The listing builds one solid part. Answer for the finished solid, in the listing's coordinates (mm). Round coordinates to 2 decimals unless told otherwise and drop trailing zeros. Loops run counter-clockwise (first coordinate to the right, second up) from the corner with the lowest first, then second, coordinate; pieces in that order, holes last. Notation, with made-up numbers: M -37,41 L 8,41 A15 cw 8,45 Z; hole C 80.5,76 d11. An arc over 180 degrees is marked long. Answer as a JSON object with one key per item and string values.
```python
from build123d import *

# Parameters (mm, degrees)
CORTAR_EXTRUIR1_DEPTH      = 11.998522628
CORTAR_EXTRUIR1_DEPTH_BACK = 11.998522628
CROQUIS2_R                 = 3
CORTAR_EXTRUIR2_DEPTH      = 11.998522628
CORTAR_EXTRUIR2_DEPTH_BACK = 11.998522628
CROQUIS3_W                 = 1.096650784
CROQUIS3_H                 = 12.7
REDONDEO1_R                = 0.25
CHAFL_N1_SIZE              = 0.5


with BuildPart() as part:
    # Croquis1 → Revolución1 (revolve)
    with BuildSketch(Plane.XY):
        with BuildLine():
            Line((0, 6.35), (0, -6.35))
            ThreePointArc((0, -6.35), (-6.35, 0), (0, 6.35))
        make_face()
    revolve(axis=Axis((0, 6.35, 0), (0, -1, 0)))

    # Croquis2 → Cortar-Extruir1 (cut, two sides: drawn at the far end of the back side and taken through both)
    with BuildSketch(Plane.XY.offset(-CORTAR_EXTRUIR1_DEPTH_BACK)):
        with Locations(Location((0, 0, 0), (0, 0, 180))):
            Circle(CROQUIS2_R)
    extrude(amount=CORTAR_EXTRUIR1_DEPTH + CORTAR_EXTRUIR1_DEPTH_BACK, mode=Mode.SUBTRACT)

    # Croquis3 → Cortar-Extruir2 (cut, two sides: drawn at the far end of the back side and taken through both)
    with BuildSketch(Plane(origin=(0, 0, 0), x_dir=(0, 0, -1), z_dir=(1, 0, 0)).offset(-CORTAR_EXTRUIR2_DEPTH_BACK)):
        with Locations((5.048325392, 0)):
            Rectangle(CROQUIS3_W, CROQUIS3_H)
        with Locations((-5.048325392, 0)):
            Rectangle(CROQUIS3_W, CROQUIS3_H)
    extrude(amount=CORTAR_EXTRUIR2_DEPTH + CORTAR_EXTRUIR2_DEPTH_BACK, mode=Mode.SUBTRACT)

    # Redondeo1
    redondeo1_edges = [part.edges().sort_by_distance(p)[0] for p in [
        (0, -4.480234369, 4.5),
        (0, 4.480234369, -4.5),
    ]]
    fillet(redondeo1_edges, radius=REDONDEO1_R)

    # Chaflán1
    chafl_n1_edges = [part.edges().sort_by_distance(p)[0] for p in [
        (3, 0, 4.5),
        (3, 0, -4.5),
    ]]
    chamfer(chafl_n1_edges, length=CHAFL_N1_SIZE)


solid = part.part
```
Item 1: The part is cut by section B-B (x = 5.75). Give the vertices of the cut face in (y, z), then the cut area to 3 significant figures.
Values follow:
{"outline": "C 0,0 d5.39", "area": "22.8 mm^2"}
Item 2: The part is cut by section D-D (x = -5.25). Give the vertices of the cut face in (y, z).
Values follow:
{"outline": "C 0,0 d7.14"}
Item 3: The part is cut by section A-A (z = 1.25). Give the vertices of the cut face in (x, y).
Values follow:
{"outline": "C 0,0 d12.45; hole C 0,0 d6"}
Item 4: The part is cut by section C-C (z = -0.75). Give the vertices of the cut face in (x, y).
Values follow:
{"outline": "C 0,0 d12.61; hole C 0,0 d6"}
Item 5: Straight lines are drawn through the part: line 1 (Y direction, x = 0, z = 0.75); line 2 (X direction, y = 1, z = 1.75); line 3 (X direction, y = 2.5, z = 2.25). For each, find the intervals that lie inside material, in ascending order.
Values follow:
{"line 1": "-6.31 to -3, 3 to 6.31", "line 2": "-6.02 to -2.83, 2.83 to 6.02", "line 3": "-5.39 to -1.66, 1.66 to 5.39"}
Item 6: Flat-ended cylindrical pins translate along their axes: P1, Ø3, axis at x = -5, z = 3, coming from the +Y side; P2, Ø1.5, axis at x = -1, z = -3, coming from the +Y side; P3, Ø2, axis at x = -5, z = 1.5, coming from the +Y side. Find the tip coordinate at first contact, or state that the pin passes through.
Values follow:
{"P1": "y = 4.64", "P2": "y = 5.87", "P3": "y = 4.74"}
Item 7: Determine the mould class of faces 1 (the face through (-4, 0, 4.5)), 2 (the face through (-2.86, -0.9, -0.06)) for opening direction X: released by +X, released by -X, zero draft, split by the parting line, or undercut.
Values follow:
{"face 1": "zero draft", "face 2": "undercut"}
